The model under review builds one solid part; all positions refer to its coordinate system, in mm. Face numbers are marked on the shaded views. Coordinates: 2 decimals unless noted, no trailing zeros. Order: outer loops, then holes, each group sorted by start corner. A loop starts at its lowest first (then second) coordinate and runs counter-clockwise, first axis right, second up. Notation, with made-up numbers: (26, 33.5) -> (50, 33.5) arc R19 cw to (50, 63.5) -> close; hole circle Ø1 at (73.5, 6). An arc over 180 degrees is marked (long way). Answer as CSV lines item,"result". Start each with the question number.
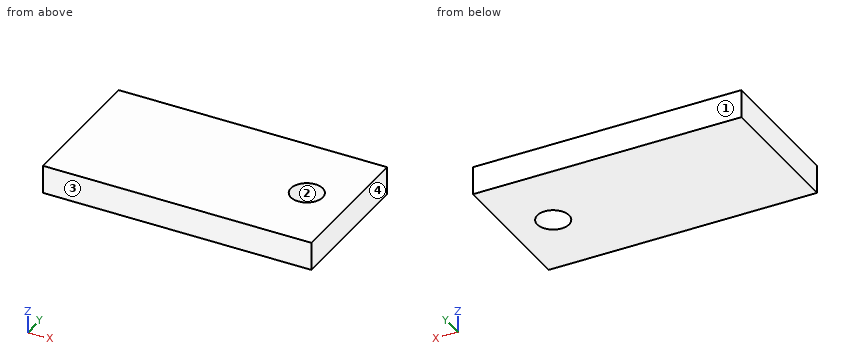
from build123d import *

# Parameters (mm, degrees)
CYLINDER098_R     = 1.13
CYLINDER098_DEPTH = 10
BOX_W             = 19
BOX_H             = 10
BOX_DEPTH         = 2


with BuildPart() as cylinder098:
    # Cylinder098 → Cylinder098 (new body)
    with BuildSketch(Plane(origin=(6.5, -83, 0), x_dir=(1, 0, 0), z_dir=(0, 0, 1))):
        Circle(CYLINDER098_R)
    extrude(amount=CYLINDER098_DEPTH)


with BuildPart() as obj1:
    # Box → Box (new body)
    with BuildSketch(Plane(origin=(-9.5, -88, 0), x_dir=(1, 0, 0), z_dir=(0, 0, 1))):
        with Locations((9.5, 5)):
            Rectangle(BOX_W, BOX_H)
    extrude(amount=BOX_DEPTH)

    # Cut018: cut Cylinder098
    add(cylinder098.part, mode=Mode.SUBTRACT)


with BuildPart() as obj1_1:
    # Cut018 placement: moved
    add(obj1.part.moved(Location((0, 0, 110))))


solid = obj1_1.part
1) Consider section C-C (z = 110.65). Give the boundary of the cut face in (x, y), plus the area to 3 significant figures.
2) Consider section B-B (y = -83). Give the boundary of the cut face in (x, z).
3) Mouldability with a two-part tool opening along Y and no side actions: class the marked faces 1, 2, 3 and 4 as released by +Y, released by -Y, zero draft, split by the parting line, or undercut.
4) Consider section A-A (x = 6.5). Give the boundary of the cut face in (y, z).
5) Wall thickness on L1, parallel to X at y = -83, z = 110.45; L2, parallel to Y at x = 6.5, z = 111.4; L3, parallel to X at y = -83.5, z = 111.6: over which ranges is each line inside the solid? List them lowest first. Write a range as [from, to].
Result:
1,outline,"(-9.5, -88) -> (9.5, -88) -> (9.5, -78) -> (-9.5, -78) -> close; hole circle Ø2.26 at (6.5, -83)"
1,area,"186 mm2"
2,outline,"(-9.5, 110) -> (5.37, 110) -> (5.37, 112) -> (-9.5, 112) -> close; (7.63, 110) -> (9.5, 110) -> (9.5, 112) -> (7.63, 112) -> close"
3,face 1,"released by +Y"
3,face 2,"undercut"
3,face 3,"released by -Y"
3,face 4,"zero draft"
4,outline,"(-88, 110) -> (-84.13, 110) -> (-84.13, 112) -> (-88, 112) -> close; (-81.87, 110) -> (-78, 110) -> (-78, 112) -> (-81.87, 112) -> close"
5,L1,"[-9.5, 5.37], [7.63, 9.5]"
5,L2,"[-88, -84.13], [-81.87, -78]"
5,L3,"[-9.5, 5.49], [7.51, 9.5]"
